Can you work these out from the model? Positions are in its coordinate system, mm. A direction names the side the tool comes from. Give positions to 0.01 mm unless a question says otherwise; leave off trailing zeros. Write each loop counter-clockwise with the first axis right and the second up, starting at its lowest first coordinate (ties: lowest second). Pieces come first, ordered by that corner, then holes.
1. I'm going to push flat-ended pins straight in: pin 1 (5 mm diameter, centred on x = 16.5, z = 11.5, fed in from -Y); pin 2 (6 mm diameter, centred on x = 25.5, y = -4, fed in from -Z); pin 3 (6 mm diameter, centred on x = 19, y = 12, fed in from +Z). Where does each tip first touch, or does it pass through?
2. If I drill on probe 1 along Y at (x, z) = (11.25, 0); probe 2 along X at (y, z) = (-4, -8.5); probe 3 along Z at (x, y) = (20, 2), over which ranges is the centre line in solid material (lowest first)?
3. Suppose I cut it at A-A (x = 8.5). Please give me the cut outline in (y, z).
4. On a 3-axis mill with a long thin cutter (end or side, diameter ignored), from which of +Z, -Z, +X, -X, +Y, -Y can I reach the whole of each face in a straight line? I mean faces 1 (the cylindrical face through (8.1, 8.54, -1.9)), 2 (the conical face through (0.326, -7.749, 13.498)), 3 (the flat face through (16, 0.1, 14.7)). Say none if no direction works.
5. Suppose I cut it at B-B (x = 18.25). Please give me the cut outline in (y, z).
```python
from build123d import *

# Parameters (mm, degrees)
BASENUT_DEPTH = 16
DOMEFILLET_R  = 1


with BuildPart() as part:
    # BaseNutSke → BaseNut (new body)
    with BuildSketch(Plane(origin=(0, 0, 0), x_dir=(0, 0, -1), z_dir=(1, 0, 0))):
        Polygon((15, 8.660254038), (15, -8.660254038), (0, -17.320508076), (-15, -8.660254038), (-15, 8.660254038), (0, 17.320508076), align=None)
    extrude(amount=BASENUT_DEPTH)

    # DomeSke → Dome (revolve)
    with BuildSketch(Plane.XY):
        with BuildLine():
            Line((29, 0), (27.4, 0))
            ThreePointArc((27.4, 0), (23.914570696, 8.414570696), (15.5, 11.9))
            Line((15.5, 11.9), (0, 11.9))
            Line((0, 11.9), (0, 13.5))
            Line((0, 13.5), (15.5, 13.5))
            ThreePointArc((15.5, 13.5), (25.045941546, 9.545941546), (29, 0))
        make_face()
    revolve(axis=Axis((0, 0, 0), (1, 0, 0)))

    # Sketch4 → DoubleChamfer (revolve, cut)
    with BuildSketch(Plane.XY):
        Polygon((0, 15), (2.783121635, 19.820508076), (13.216878365, 19.820508076), (16, 15), (18, 15), (18, 30), (-2, 30), (-2, 15), align=None)
    revolve(axis=Axis((0, 0, 0), (1, 0, 0)), mode=Mode.SUBTRACT)

    # TapDriSke → TapDrill (revolve, cut)
    with BuildSketch(Plane.XY, mode=Mode.PRIVATE) as tapdrill_sk:
        Polygon((0, 8.75), (21.4, 8.75), (26.657530416, 0), (0, 0), align=None)
    revolve(tapdrill_sk.sketch.rotate(Axis((0, 0, 0), (1, 0, 0)), 90), axis=Axis((0, 0, 0), (1, 0, 0)), mode=Mode.SUBTRACT)

    # EndChamferSketch → EndChamfer (revolve, cut)
    with BuildSketch(Plane.XY, mode=Mode.PRIVATE) as endchamfer_sk:
        Polygon((-0.0746, 10), (0.0254, 10), (0.988185365, 8.625), (-0.0746, 8.625), align=None)
        Polygon((15.9746, 10), (16.1, 10), (16.1, 8.625), (15.011814635, 8.625), align=None)
    revolve(endchamfer_sk.sketch.rotate(Axis((0, 0, 0), (-1, 0, 0)), 90), axis=Axis((0, 0, 0), (-1, 0, 0)), mode=Mode.SUBTRACT)

    # DomeFillet
    domefillet_edges = [part.edges().sort_by_distance(p)[0] for p in [
        (16, -13.490737563, 0),
    ]]
    fillet(domefillet_edges, radius=DOMEFILLET_R)


solid = part.part
```
Checks:
1. pin 1: stops at y = -12.09
1. pin 2: stops at z = -11.04
1. pin 3: stops at z = 9.59
2. probe 1: y = -17.32 to -8.75, 8.75 to 17.32
2. probe 2: x = 0.45 to 15.55, 22.8 to 25.2
2. probe 3: z = -12.57 to -10.83, 10.83 to 12.57
3. outline: (-17.32, 0) - (-8.66, -15) - (8.66, -15) - (17.32, 0) - (8.66, 15) - (-8.66, 15) - close; hole circle Ø17.5 at (0, 0)
4. face 1: -X
4. face 2: +Z, -X, -Y
4. face 3: +X
5. outline: circle Ø26.43 at (0, 0); hole circle Ø23.16 at (0, 0)
